Can you work these out from the model? Positions are in its coordinate system, mm. Face numbers are marked on the shaded views. A direction names the side the tool comes from. Round coordinates to 2 decimals unless told otherwise and drop trailing zeros. Order: outer loops, then holes, each group sorted by start corner. A loop starts at its lowest first (then second) coordinate and runs counter-clockwise, first axis right, second up. Notation, with made-up numbers: (58, -26) - (69, -26) arc R18 ccw to (69, 2) - close; hole circle Ø9 at (24, 82.5). An arc over 180 degrees is marked (long way). Write item = value, one per line.
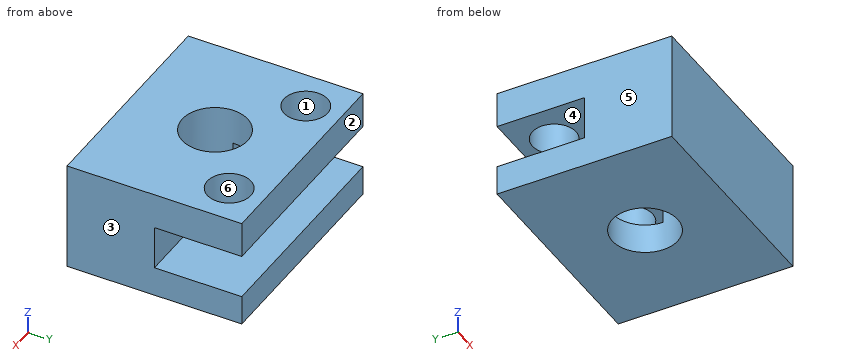
from build123d import *

# Parameters (mm, degrees)
F0_W     = 100
F0_H     = 80
F0_R     = 15
F1_DEPTH = 50
F3_W     = 122.5489005446
F3_H     = 20
F4_DEPTH = 40
F5_R     = 10
F6_DEPTH = 16.3678393885


# Not quite as in the source:
# - a pattern or mirror of a feature is missing from the dataset's text; its kind, count and spacing are read off the source's solid


with BuildPart() as f1:
    # F0 (on Top) → F1 (new body)
    with BuildSketch(Plane.XY):
        Rectangle(F0_W, F0_H)
        Circle(F0_R, mode=Mode.SUBTRACT)
    extrude(amount=F1_DEPTH)

    # F3 (on offset) → F4 (cut)
    with BuildSketch(Plane.XZ.offset(-40)):
        with Locations((0.9837634861, 23.6321606115)):
            Rectangle(F3_W, F3_H)
    extrude(amount=F4_DEPTH, mode=Mode.SUBTRACT)

    # F5 (on face) → F6 (cut, through all)
    with BuildSketch(Plane.XY.offset(50)):
        with Locations((31.620990485, 24.0319501609)):
            Circle(F5_R)
    f6 = extrude(amount=-F6_DEPTH, mode=Mode.SUBTRACT)

    # F6_copies: F6 across plane
    add(f6.mirror(Plane(origin=(0, 0, 0), x_dir=(0, 0, -1), z_dir=(-1, 0, 0))), mode=Mode.SUBTRACT)


solid = f1.part
(1) If we section it at A-A (x = 0): Write out the boundary of the cut face in (y, z), plus the area to 3 significant figures.
Computed:
outline = (-40, 0) - (-15, 0) - (-15, 50) - (-40, 50) - close; (15, 0) - (40, 0) - (40, 13.63) - (15, 13.63) - close; (15, 33.63) - (40, 33.63) - (40, 50) - (15, 50) - close
area = 2,000 mm^2
(2) If we section it at B-B (z = 7): Write out the boundary of the cut face in (x, y).
Computed:
outline = (-50, -40) - (50, -40) - (50, 40) - (-50, 40) - close; hole circle Ø30 at (0, 0)
(3) If I drill on line 1 (X direction, y = 24, z = 40.5); line 2 (Y direction, x = 0, z = 11); line 3 (Z direction, x = 21.5, y = 27), over which ranges is the centre line in solid material (lowest first)? Write a range as from..to.
Computed:
line_1 = -50..-41.62, -21.62..21.62, 41.62..50
line_2 = -40..-15, 15..40
line_3 = 0..13.63, 33.63..50
(4) Thinking about a two-plate mould opening in X: for the marked faces 1, 2 and 3, which applies, +X half, -X half, draft (parallel to the pull), parting line (faces both ways), or undercut?
Computed:
face_1 = undercut
face_2 = draft
face_3 = +X half
(5) If we section it at C-C (x = -27.5): Write out the boundary of the cut face in (y, z), plus the area to 3 significant figures.
Computed:
outline = (-40, 0) - (40, 0) - (40, 13.63) - (0, 13.63) - (0, 33.63) - (14.92, 33.63) - (14.92, 50) - (-40, 50) - close; (33.14, 33.63) - (40, 33.63) - (40, 50) - (33.14, 50) - close
area = 2,900 mm^2
(6) On a 3-axis mill with a long thin cutter (end or side, diameter ignored), from which of +Z, -Z, +X, -X, +Y, -Y can I reach the whole of each face in a straight line? I mean the marked faces 4, 5 and 6. Say none if no direction works.
Computed:
face_4 = +X, -X, +Y
face_5 = +Z, -Z, -X, +Y, -Y
face_6 = +Z
(7) If we section it at D-D (y = 30): Write out the boundary of the cut face in (x, z), plus the area to 3 significant figures.
Computed:
outline = (-50, 0) - (50, 0) - (50, 13.63) - (-50, 13.63) - close; (-50, 33.63) - (-39.64, 33.63) - (-39.64, 50) - (-50, 50) - close; (-23.6, 33.63) - (23.6, 33.63) - (23.6, 50) - (-23.6, 50) - close; (39.64, 33.63) - (50, 33.63) - (50, 50) - (39.64, 50) - close
area = 2,470 mm^2
(8) Will these pins go through, and if not, where does the flat tip stop? P1, Ø6, axis at x = -35, z = 20, coming from the +Y side; P2, Ø1, axis at x = 37.5, y = 19, coming from the +Z side.
Computed:
P1 = 0
P2 = 13.63
